```python
from build123d import *

# Parameters (mm, degrees)
SKETCH1_R           = 170
BOSS_EXTRUDE1_DEPTH = 22.5
SKETCH2_R           = 170.69
BOSS_EXTRUDE2_DEPTH = 2
CUT_EXTRUDE1_START  = -10
SKETCH3_R           = 131.78
SKETCH3_R_2         = 60
CUT_EXTRUDE1_DEPTH  = 233.632236523
SKETCH4_R           = 30
CUT_EXTRUDE2_DEPTH  = 247.315148133
CUT_EXTRUDE3_DEPTH  = 247.315148133


with BuildPart() as part:
    # Sketch1 → Boss-Extrude1 (new, symmetric)
    with BuildSketch(Plane(origin=(0, 0, 0), x_dir=(1, 0, 0), z_dir=(0, 1, 0))):
        with Locations(Location((0, 0, 0), (0, 0, 90))):
            Circle(SKETCH1_R)
    extrude(amount=BOSS_EXTRUDE1_DEPTH, both=True)

    # Sketch2 → Boss-Extrude2 (add)
    with BuildSketch(Plane(origin=(0, 22.5, 0), x_dir=(1, 0, 0), z_dir=(0, 1, 0))):
        with Locations(Location((0, 0, 0), (0, 0, 270))):
            Circle(SKETCH2_R)
    boss_extrude2 = extrude(amount=BOSS_EXTRUDE2_DEPTH)

    # Mirror1: Boss-Extrude2 across plane
    add(boss_extrude2.mirror(Plane.ZX))

    # Sketch3 → Cut-Extrude1 (cut, through all)
    with BuildSketch(Plane(origin=(0, 0, 0), x_dir=(1, 0, 0), z_dir=(0, 1, 0)).offset(CUT_EXTRUDE1_START)):
        with Locations(Location((0, 0, 0), (0, 0, 270))):
            Circle(SKETCH3_R)
        with Locations(Location((0, 0, 0), (0, 0, 270))):
            Circle(SKETCH3_R_2, mode=Mode.SUBTRACT)
    cut_extrude1 = extrude(amount=-CUT_EXTRUDE1_DEPTH, mode=Mode.SUBTRACT)

    # Mirror3: Cut-Extrude1 across plane
    add(cut_extrude1.mirror(Plane.ZX), mode=Mode.SUBTRACT)

    # Sketch4 → Cut-Extrude2 (cut, through all)
    with BuildSketch(Plane.XZ.offset(24.5)):
        with Locations(Location((0, 0, 0), (0, 0, 270))):
            Circle(SKETCH4_R)
    extrude(amount=-CUT_EXTRUDE2_DEPTH, mode=Mode.SUBTRACT)

    # Sketch5 → Cut-Extrude3 (cut, through all)
    with BuildSketch(Plane.XZ.offset(24.5)):
        with BuildLine():
            Line((-9, 34.650252524), (-9, 18.069809638))
            Line((-9, 18.069809638), (9, 18.069809638))
            Line((9, 18.069809638), (9, 34.650252524))
            ThreePointArc((9, 34.650252524), (0, 35.8), (-9, 34.650252524))
        make_face()
    extrude(amount=-CUT_EXTRUDE3_DEPTH, mode=Mode.SUBTRACT)


solid = part.part
```
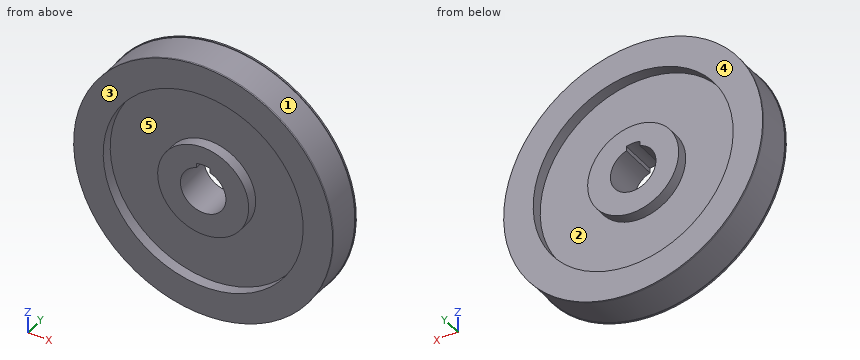
The model under review builds one solid part; all positions refer to its coordinate system, in mm. Face numbers are marked on the shaded views. A direction names the side the tool comes from. Round coordinates to 2 decimals unless told otherwise and drop trailing zeros. Order: outer loops, then holes, each group sorted by start corner. A loop starts at its lowest first (then second) coordinate and runs counter-clockwise, first axis right, second up. Notation, with made-up numbers: (64, 9) -> (115, 9) arc R11 cw to (115, 22) -> close; hole circle Ø9 at (59, -30). An arc over 180 degrees is marked (long way). One line per item, written item: value. Start each with the question number.
Q1. Machinability: for the marked faces 4 and 5, which of the approach directions +Z, -Z, +X, -X, +Y, -Y give a long, thin tool a straight path to every point of the face, cutting with its end or side? Answer none if there is none.
Q2. Take a section at A-A (y = 17). Write out the cut boundary in (x, z).
Q3. Wall thickness on line 1 (X direction, y = -14, z = 0); line 2 (X direction, y = -21.5, z = 48.5); line 3 (X direction, y = 21, z = 25.5): over which ranges is each line inside the solid? List them lowest first.
Q4. Take a section at D-D (x = -36.5). Write out the cut boundary in (y, z).
Q5. Clearance check with flat-ended pins moving along their axes: pin 1 Ø5 at (y, z) = (9.5, 47) entering from +X; pin 2 Ø8 at (y, z) = (2.5, 46.5) entering from -X; pin 3 Ø5 at (y, z) = (6, 32.5) entering from +X. State where each tip first meets the part, or that it passes through.
Q6. Mouldability with a two-part tool opening along X and no side actions: class the marked faces 1, 2 and 3 as released by +X, released by -X, zero draft, split by the parting line, or undercut.
Reported:
1. face 4: +Z, -Z, +X, -X, +Y
1. face 5: -Y
2. outline: circle Ø340 at (0, 0); circle Ø120 at (0, 0); hole circle Ø263.56 at (0, 0); hole (-9, 28.62) arc R30 ccw (long way) to (9, 28.62) -> (9, 34.65) arc R35.8 ccw to (-9, 34.65) -> close
3. line 1: x = -170 to -131.78, -60 to -30, 30 to 60, 131.78 to 170
3. line 2: x = -162.93 to -122.53, -35.32 to 35.32, 122.53 to 162.93
3. line 3: x = -168.08 to -129.29, -54.31 to -15.8, 15.8 to 54.31, 129.29 to 168.08
4. outline: (-24.5, -166.74) -> (-22.5, -166.74) -> (-22.5, -166.04) -> (22.5, -166.04) -> (22.5, -166.74) -> (24.5, -166.74) -> (24.5, -126.62) -> (10, -126.62) -> (10, -47.62) -> (24.5, -47.62) -> (24.5, 47.62) -> (10, 47.62) -> (10, 126.62) -> (24.5, 126.62) -> (24.5, 166.74) -> (22.5, 166.74) -> (22.5, 166.04) -> (-22.5, 166.04) -> (-22.5, 166.74) -> (-24.5, 166.74) -> (-24.5, 126.62) -> (-10, 126.62) -> (-10, 47.62) -> (-24.5, 47.62) -> (-24.5, -47.62) -> (-10, -47.62) -> (-10, -126.62) -> (-24.5, -126.62) -> close
5. pin 1: stops at x = 164.07
5. pin 2: stops at x = -164.6
5. pin 3: stops at x = 167.33
6. face 1: split by the parting line
6. face 2: undercut
6. face 3: zero draft
